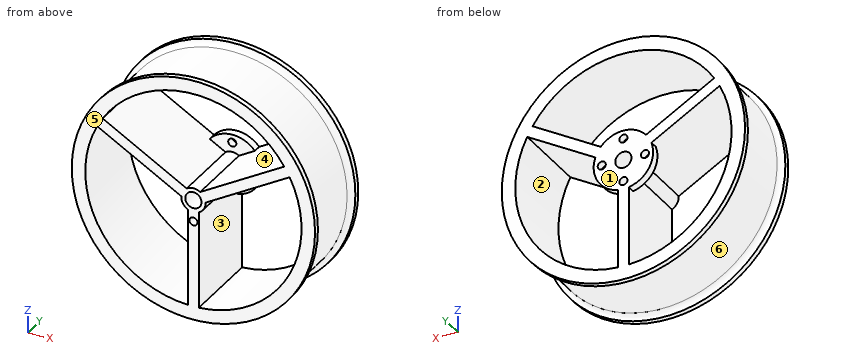
Autodesk Inventor part; units mm, degrees
ref_plane "YZ Plane" through (0, 0, 0) normal (1, 0, 0) x (0, 1, 0)
ref_plane "XZ Plane" through (0, 0, 0) normal (0, 1, 0) x (-1, 0, 0)
ref_plane "XY Plane" through (0, 0, 0) normal (0, 0, 1) x (1, 0, 0)
sketch "Эскиз1" plane through (0, 0, 0) normal (0, 0, 1) x (1, 0, 0)
  line L0 (0, 0) -> (40, 0)
  line L1 (0, 0) -> (0, 10)
  line L2 (40, 0) -> (40, -15) construction
  line L3 (40, -15) -> (45, -15)
  line L4 (45, 15) -> (40, 15)
  line L5 (40, 15) -> (40, -15)
  line L6 (40, 15) -> (40, 13) construction
  line L7 (40, 13) -> (45, 13) construction
  line L8 (40, -15) -> (40, -13) construction
  line L9 (40, -13) -> (45, -13) construction
  line L10 (45, -13) -> (45, -11) construction
  line L11 (45, -11) -> (45, -9) construction
  arc A0 (43, -11) -> (45, -13) centre (45, -11) ccw
  arc A1 (45, 13) -> (43, 11) centre (45, 11) ccw
  line L12 (43, 11) -> (43, -11)
  line L13 (45, -15) -> (45, -13)
  line L14 (45, 13) -> (45, 15)
  dimension "d0" = 40
  dimension "d1" = 10
  dimension "d2" = 15
  dimension "d3" = 5
  dimension "d4" = 30
  dimension "d5" = 2
  dimension "d6" = 2
revolve "Вращение1" add sketch "Эскиз1" angle 360 about axis through (0, 0, 0) along (0, 1, 0)
sketch "Эскиз7" plane through (0, 15, 0) normal (0, 1, 0) x (1, 0, 0)
  circle A0 centre (0, 0) radius 11
  dimension "d29" = 22
extrude "Выдавливание5" add sketch "Эскиз7" against normal blind 3
sketch "Эскиз8" plane through (0, 15, 0) normal (0, 1, 0) x (1, 0, 0)
  circle A0 centre (0, 0) radius 3
  circle A1 centre (0, 0) radius 4.5
  dimension "d32" = 6
  dimension "d33" = 9
extrude "Выдавливание6" cut sketch "Эскиз8" against normal blind 3 contours A0
extrude "Выдавливание7" add sketch "Эскиз8" against normal up to surface (30 mm away)
sketch "Эскиз10" plane through (0, 15, 0) normal (0, 1, 0) x (1, 0, 0)
  line L0 (0, 0) -> (8, 0) construction
  circle A0 centre (8, 0) radius 1.5
  circle A1 centre (0, 0) radius 3 construction
  circle A2 centre (0, 8) radius 1.5
  circle A3 centre (-8, 0) radius 1.5
  circle A4 centre (0, -8) radius 1.5
  dimension "d38" = 8
  dimension "d39" = 3
  dimension "d42" = 360
extrude "Выдавливание8" cut sketch "Эскиз10" against normal blind 3
sketch "Эскиз11" plane through (0, -15, 0) normal (0, -1, 0) x (1, 0, 0)
  circle A0 centre (0, 0) radius 3
  circle A1 centre (0, 0) radius 4.5
  circle A2 centre (0, 0) radius 45
  circle A3 centre (0, 0) radius 40
  line L0 (0, -4.5) -> (0, -40) construction
  circle A4 centre (0, 0) radius 40 construction
  line L1 (-2, -39.95) -> (-2, -4.0311)
  line L2 (2, -4.0311) -> (2, -39.95)
  line L3 (1.8638, -39.9566) -> (-1.9134, -4.073) construction
  line L4 (-1.8638, -39.9566) -> (1.9134, -4.073) construction
  circle A5 centre (0, -8) radius 1.5
  arc A6 (-2, -39.95) -> (2, -39.95) centre (0, 0) ccw
  arc A7 (-2, -4.0311) -> (1.9134, -4.073) centre (0, 0) ccw
  point P0 (0, -22.25)
extrude "Выдавливание9" add sketch "Эскиз11" against normal up to surface (30 mm away) contours A1 L2 A3 L1 | A5 picked at (0.0603, -29.826)
pattern_circular "Круговой массив1" count 3 over 360 about axis through (0, 15, 0) along (0, -1, 0) of "Выдавливание9"
sketch "Эскиз12" plane through (0, 15, 0) normal (0, 1, 0) x (1, 0, 0)
  circle A0 centre (8, 0) radius 1.5
  circle A1 centre (0, 0) radius 3
  circle A2 centre (8, 0) radius 1.5
  circle A3 centre (0, 8) radius 1.5
  circle A4 centre (-8, 0) radius 1.5
  circle A5 centre (0, -8) radius 1.5
  dimension "d55" = 360
extrude "Выдавливание10" cut sketch "Эскиз12" against normal up to next contours A3
properties part number "Wheel"
Model file for the job. Use its own axes, mm. Face numbers are marked on the shaded views. A direction names the side the tool comes from. Give positions to 0.01 mm unless a question says otherwise; leave off trailing zeros. Loops run counter-clockwise (first coordinate to the right, second up) from the corner with the lowest first, then second, coordinate; pieces in that order, holes last.
1) Saw through at B-B (y = -4.75). Write the cut outline in (x, z), plus the area to 3 significant figures.
2) Saw through at A-A (x = 0). Count the separate pieces of the cut face and the enclosed holes in it, plus the area to 3 significant figures.
3) Tool access for the marked faces 1, 2 and 3: list every direction of +Z, -Z, +X, -X, +Y, -Y with a clear straight run to the whole face (end or side of a thin tool).
4) Pull direction X, two halves, no side cores. Call the marked faces 4, 5 and 6: +X half, -X half, draft (parallel to the pull), parting line (faces both ways), or undercut.
5) Flat gauge pins, fed straight in: pin 1 Ø3.5 at (x, z) = (-8, 0) entering from -Y; pin 2 Ø4.5 at (x, z) = (-6, -0.5) entering from -Y; pin 3 Ø5 at (x, y) = (-5, -1.5) entering from -Z; pin 4 Ø5 at (x, y) = (9, -3.5) entering from -Z. Where does each tip first touch, or does it go through?
6) Wall check: line 1 (Z direction, x = 0, y = -5); line 2 (X direction, y = 13.15, z = 0); line 3 (Z direction, x = 0, y = 13.1). Give the ranges that are in metal, low to high.
Answer block:
1. outline: circle Ø86 at (0, 0); hole (-35.6, 18.24) arc R40 ccw to (-2, -39.95) - (-2, -4.03) arc R4.5 cw to (-4.49, 0.28) - close; hole (-33.6, 21.71) - (-2.49, 3.75) arc R4.5 cw to (2.49, 3.75) - (33.6, 21.71) arc R40 ccw to start; hole circle Ø6 at (0, 0); hole circle Ø3 at (0, -8); hole (2, -39.95) arc R40 ccw to (35.6, 18.24) - (4.49, 0.28) arc R4.5 cw to (2, -4.03) - close
1. area: 1,240 mm2
2. separate pieces: 5
2. enclosed holes: 0
2. area: 1,270 mm2
3. face 1: +Z, -Z, +X, -X, +Y
3. face 2: +Y, -Y
3. face 3: -Y
4. face 4: undercut
4. face 5: draft
4. face 6: parting line
5. pin 1: stops at y = 12
5. pin 2: stops at y = -15
5. pin 3: stops at z = -42.93
5. pin 4: stops at z = -42.51
6. line 1: z = -43 to -9.5, -6.5 to -3, 3 to 4.5, 40 to 43
6. line 2: x = -45 to -40, -11 to -9.5, -6.5 to -3, 3 to 6.5, 9.5 to 11, 40 to 45
6. line 3: z = -45 to -9.5, -6.5 to -3, 3 to 6.5, 9.5 to 11, 40 to 45
